Here's how the part is built. I have some questions about the finished solid (model axes, mm). Face numbers are marked on the shaded views. A direction names the side the tool comes from. Coordinates: 2 decimals unless noted, no trailing zeros. Write each loop counter-clockwise with the first axis right and the second up, starting at its lowest first coordinate (ties: lowest second). Pieces come first, ordered by that corner, then holes.
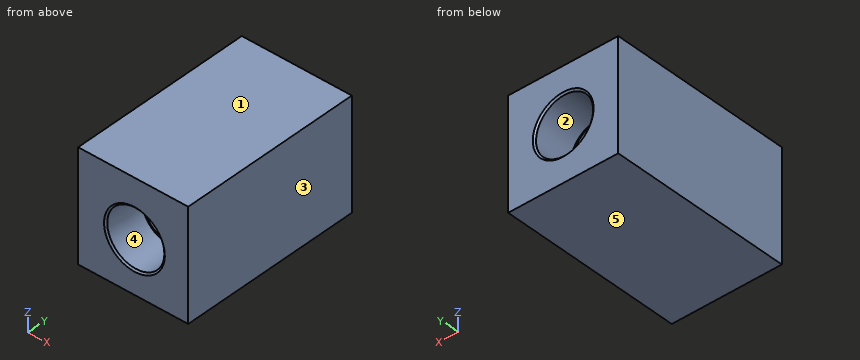
```python
from build123d import *

# Parameters (mm, degrees)
SKETCH_1_W         = 38.1
SKETCH_1_H         = 38.1
EXTRUDE_1_DEPTH    = 63.5
SKETCH5_R          = 5.588
CUT_EXTRUDE1_DEPTH = 69.978656119


with BuildPart() as part:
    # Sketch 1 → Extrude 1 (new body)
    with BuildSketch(Plane(origin=(0, 0, 0), x_dir=(1, 0, 0), z_dir=(0, 1, 0))):
        Rectangle(SKETCH_1_W, SKETCH_1_H)
    extrude(amount=EXTRUDE_1_DEPTH)

    # Sketch2 → 1_2 NPT Tapped Hole2 (revolve, cut)
    with BuildSketch(Plane(origin=(0, 63.5, 0), x_dir=(0, 0, 1), z_dir=(1, 0, 0))):
        Polygon((0, 0), (0, 28.004543693), (8.9281, 22.64), (8.9281, 13.57), (9.479012286, 13.57), (9.8860229, 0.532828266), (10.5210229, 0), align=None)
    revolve(axis=Axis((0, 69.85, 0), (0, -1, 0)), mode=Mode.SUBTRACT)

    # Sketch4 → 1_2 NPT Tapped Hole1 (revolve, cut)
    with BuildSketch(Plane(origin=(0.428891136, 0, -0.986449612), x_dir=(0, 0, -1), z_dir=(1, 0, 0))):
        Polygon((0, 0), (0, 28.004543693), (8.9281, 22.64), (8.9281, 13.57), (9.479012286, 13.57), (9.8860229, 0.532828266), (10.5210229, 0), align=None)
    revolve(axis=Axis((0.428891136, -6.35, -0.986449612), (0, 1, 0)), mode=Mode.SUBTRACT)

    # Sketch5 → Cut-Extrude1 (cut, through all)
    with BuildSketch(Plane(origin=(0, 63.5, 0), x_dir=(1, 0, 0), z_dir=(0, 1, 0))):
        with Locations(Location((0, 0, 0), (0, 0, 270))):
            Circle(SKETCH5_R)
    extrude(amount=-CUT_EXTRUDE1_DEPTH, mode=Mode.SUBTRACT)


solid = part.part
```
1) Imagine slicing it at B-B on y = 12. Please give me the cut outline in (x, z).
Values follow:
outline: (-19.05, -19.05) - (19.05, -19.05) - (19.05, 19.05) - (-19.05, 19.05) - close; hole circle Ø19.06 at (0.43, -0.99)
2) Imagine slicing it at A-A on y = 26. Please give me the cut outline in (x, z), then the cut area to 3 significant figures.
Values follow:
outline: (-19.05, -19.05) - (19.05, -19.05) - (19.05, 19.05) - (-19.05, 19.05) - close; hole circle Ø11.18 at (0, 0)
area: 1,350 mm2
3) On a 3-axis mill with a long thin cutter (end or side, diameter ignored), from which of +Z, -Z, +X, -X, +Y, -Y can I reach the whole of each face in a straight line? I mean the marked faces 4 and 5. Say none if no direction works.
Values follow:
face 4: -Y
face 5: -Z, +X, -X, +Y, -Y
4) Will these pins go through, and if not, where does the flat tip stop? pin 1 (4 mm diameter, centred on x = -6.5, z = 3, fed in from +Y); pin 2 (16 mm diameter, centred on x = 0.43, z = -0.99, fed in from -Y); pin 3 (13 mm diameter, centred on x = 0, z = 0, fed in from -Y).
Values follow:
pin 1: stops at y = 49.93
pin 2: stops at y = 23.2
pin 3: stops at y = 23.45
5) I need wall thicknesses on probe 1 along Z at (x, y) = (0, 45.25); probe 2 along X at (y, z) = (29, 0). Which ranges of each line are inside material? Lowest first, please.
Values follow:
probe 1: z = -19.05 to -8.93, 8.93 to 19.05
probe 2: x = -19.05 to -5.59, 5.59 to 19.05
6) We'd pull the mould along X, two halves only. Please class the marked faces 1, 2 and 3: pulls with the +X half, pulls with the -X half, needs draft (parallel to the pull), parting line crosses it, or undercut.
Values follow:
face 1: needs draft
face 2: undercut
face 3: pulls with the +X half
